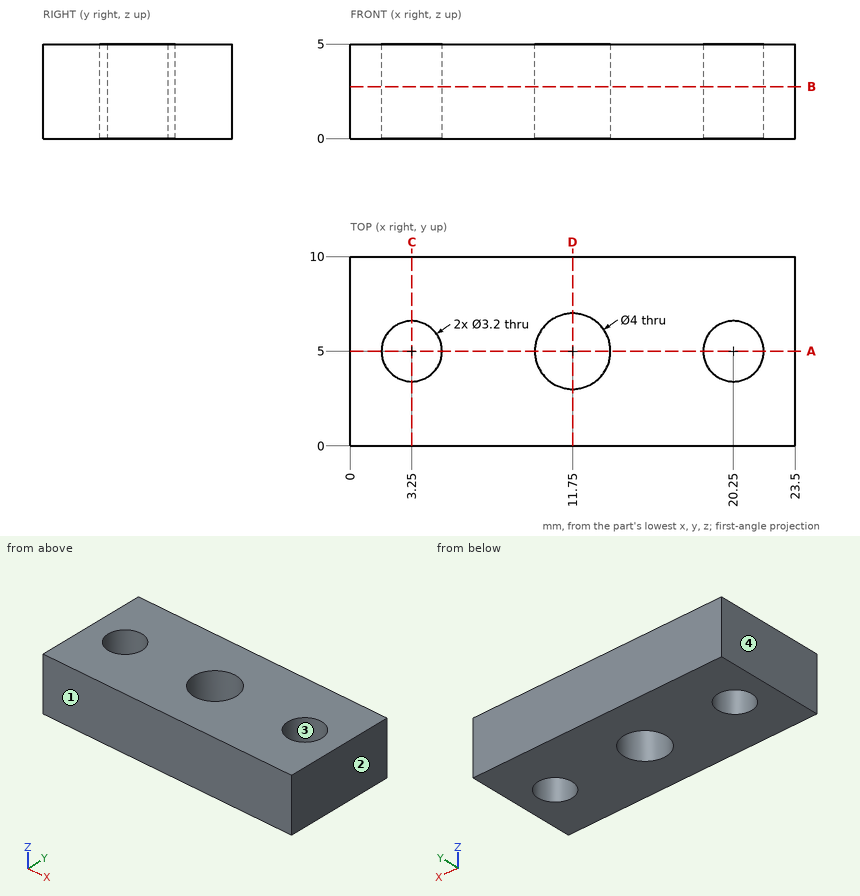
Answer from the drawing. Dimensions are ordinates in mm from the lowest x, y and z of the part. Round coordinates to 2 decimals unless told otherwise and drop trailing zeros. Loops run counter-clockwise (first coordinate to the right, second up) from the corner with the lowest first, then second, coordinate; pieces in that order, holes last. Notation, with made-up numbers: M -19,81.25 L -2,81.25 A21 cw -2,95.25 Z; hole C -7.5,52 d5. An arc over 180 degrees is marked long. One line per question, with ' | ' between items. Start each with the question number.
(1) A cutting plane is placed at B-B on z = 2.75. Write down the section's boundary in (x, y).
(2) A cutting plane is placed at C-C on x = 3.25. Write down the section's boundary in (y, z).
(3) A cutting plane is placed at D-D on x = 11.75. Write down the section's boundary in (y, z), plus the area to 3 significant figures.
(4) A cutting plane is placed at A-A on y = 5. Write down the section's boundary in (x, z).
(5) Find the intervals of material crossed by line 1 (Y direction, x = 3.25, z = 3.55); line 2 (Y direction, x = 11.75, z = 2.1); line 3 (X direction, y = 6.25, z = 2.85), in increasing order.
(6) For a pull along X with two mould halves and no side action, classify the marked faces 1, 2, 3 and 4 as released by +X, released by -X, zero draft, split by the parting line, or undercut.
Geometry check:
1) outline: M 0,0 L 23.5,0 L 23.5,10 L 0,10 Z; hole C 3.25,5 d3.2; hole C 11.75,5 d4; hole C 20.25,5 d3.2
2) outline: M 0,0 L 3.4,0 L 3.4,5 L 0,5 Z; M 6.6,0 L 10,0 L 10,5 L 6.6,5 Z
3) outline: M 0,0 L 3,0 L 3,5 L 0,5 Z; M 7,0 L 10,0 L 10,5 L 7,5 Z | area: 30.0 mm²
4) outline: M 0,0 L 1.65,0 L 1.65,5 L 0,5 Z; M 4.85,0 L 9.75,0 L 9.75,5 L 4.85,5 Z; M 13.75,0 L 18.65,0 L 18.65,5 L 13.75,5 Z; M 21.85,0 L 23.5,0 L 23.5,5 L 21.85,5 Z
5) line 1: y = 0 to 3.4, 6.6 to 10 | line 2: y = 0 to 3, 7 to 10 | line 3: x = 0 to 2.25, 4.25 to 10.19, 13.31 to 19.25, 21.25 to 23.5
6) face 1: zero draft | face 2: released by +X | face 3: undercut | face 4: released by -X
